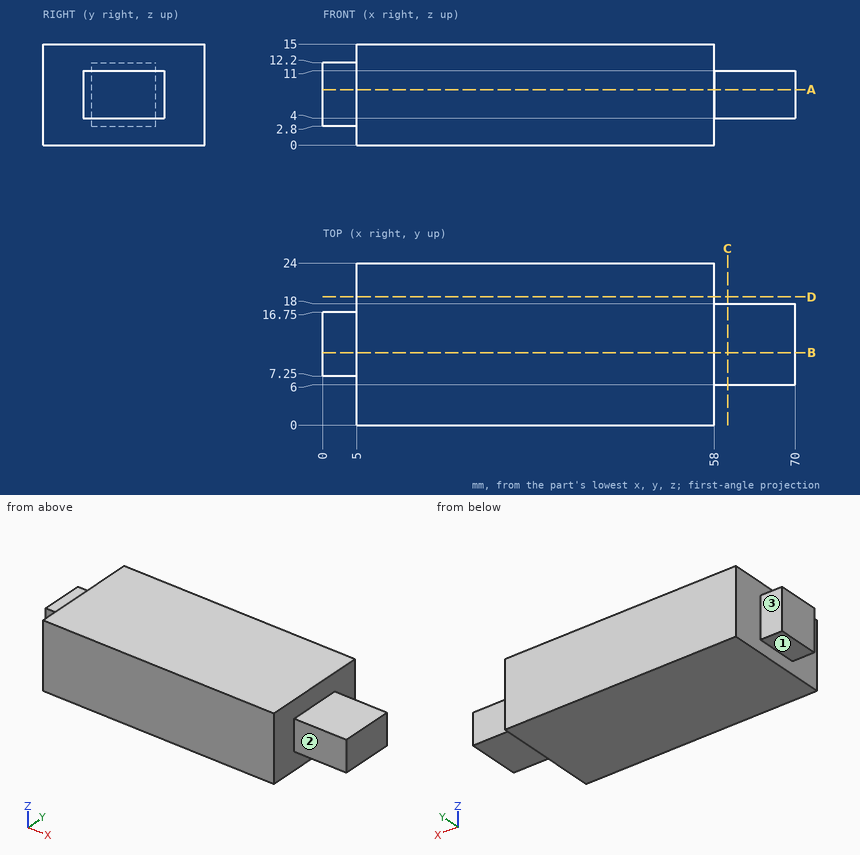
The figure shows three views and two pictorial views of one solid part (mm, origin at its lowest corner). Answer the questions. A direction names the side the tool comes from. Round coordinates to 2 decimals unless told otherwise and drop trailing zeros. Order: outer loops, then holes, each group sorted by start corner. A loop starts at its lowest first (then second) coordinate and runs counter-clockwise, first axis right, second up. Notation, with made-up numbers: M -37,59.25 L -5,59.25 A26 ccw -5,76.25 Z; hole C 37.25,15 d3. An arc over 180 degrees is marked long. Answer in a Markdown table with one row per item. Add a question column.
1) Consider line 1 along Z through (x, y) = (59.5, 13); line 2 along X through (y, z) = (16.75, 1.25); line 3 along Y through (x, z) = (67.5, 8.5). Determine where each line is inside the solid, lowest interval first. Write a range as from..to.
2) The part is cut by section A-A on z = 8.25. Determine the outline of the cut face in (x, y), plus the area to 3 significant figures.
3) Which of the six approach directions +Z, -Z, +X, -X, +Y, -Y give full straight-line access (tool end or side, diameter ignored) to the marked faces 1, 2 and 3?
4) The part is cut by section C-C on x = 60. Determine the outline of the cut face in (y, z), plus the area to 3 significant figures.
5) The part is cut by section B-B on y = 10.75. Determine the outline of the cut face in (x, z).
6) The part is cut by section D-D on y = 19. Determine the outline of the cut face in (x, z).
7) Flat-ended cylindrical pins translate along their axes: pin 1 Ø1.5 at (x, z) = (1.5, 8.5) entering from +Y; pin 2 Ø7.5 at (x, z) = (62.5, 8.5) entering from +Y; pin 3 Ø1 at (y, z) = (3.5, 5.5) entering from +X. Find the tip coordinate at first contact, or state that the pin passes through.
Findings below:
| question | item | result |
|---|---|---|
| 1 | line 1 | z = 4..11 |
| 1 | line 2 | x = 5..58 |
| 1 | line 3 | y = 6..18 |
| 2 | outline | M 0,7.25 L 5,7.25 L 5,0 L 58,0 L 58,6 L 70,6 L 70,18 L 58,18 L 58,24 L 5,24 L 5,16.75 L 0,16.75 Z |
| 2 | area | 1,460 mm² |
| 3 | face 1 | -Z, -X, +Y, -Y |
| 3 | face 2 | +Z, -Z, +X, -Y |
| 3 | face 3 | +Z, -Z, -X, +Y |
| 4 | outline | M 6,4 L 18,4 L 18,11 L 6,11 Z |
| 4 | area | 84.0 mm² |
| 5 | outline | M 0,2.8 L 5,2.8 L 5,0 L 58,0 L 58,4 L 70,4 L 70,11 L 58,11 L 58,15 L 5,15 L 5,12.2 L 0,12.2 Z |
| 6 | outline | M 5,0 L 58,0 L 58,15 L 5,15 Z |
| 7 | pin 1 | stops at y = 16.75 |
| 7 | pin 2 | stops at y = 18 |
| 7 | pin 3 | stops at x = 58 |
